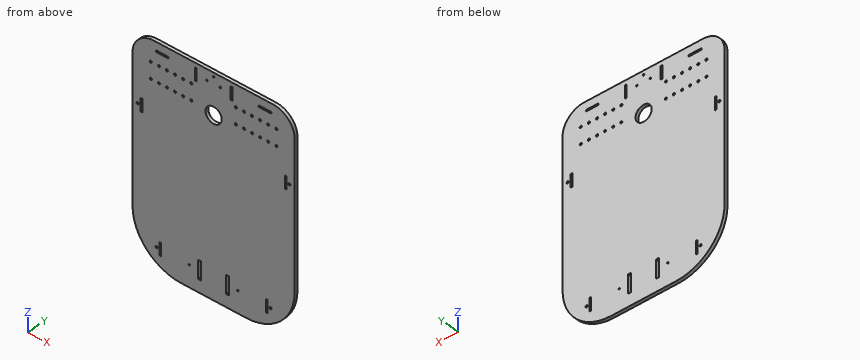
Autodesk Inventor part; units mm, degrees
ref_plane "YZ Plane" through (0, 0, 0) normal (1, 0, 0) x (0, 1, 0)
ref_plane "XZ Plane" through (0, 0, 0) normal (0, 1, 0) x (-1, 0, 0)
ref_plane "XY Plane" through (0, 0, 0) normal (0, 0, 1) x (1, 0, 0)
sketch "Sketch1" plane through (0, 0, 0) normal (0, 1, 0) x (-1, 0, 0)
  line L0 (150, 200) -> (-150, 200)
  line L1 (-150, 200) -> (-150, -200)
  line L2 (-150, -200) -> (150, -200)
  line L3 (150, -200) -> (150, 200)
  line L4 (150, 200) -> (-150, -200) construction
  line L5 (-150, 200) -> (150, -200) construction
  point P0 (0, 0)
  dimension "d0" = 300
  dimension "d1" = 400
extrude "Extrusion1" add sketch "Sketch1" along normal blind 6
sketch "Sketch2" plane through (0, 6, 0) normal (0, 1, 0) x (1, 0, 0)
  line L0 (116.2, -158) -> (86.2, -158) construction
  line L1 (86.2, -162) -> (116.2, -162) construction
  arc A0 (86.2, -158) -> (86.2, -162) centre (86.2, -160) ccw construction
  arc A1 (116.2, -162) -> (116.2, -158) centre (116.2, -160) ccw construction
  line L2 (86.2, -132) -> (116.2, -132) construction
  line L3 (116.2, -128) -> (86.2, -128) construction
  arc A2 (116.2, -132) -> (116.2, -128) centre (116.2, -130) ccw construction
  arc A3 (86.2, -128) -> (86.2, -132) centre (86.2, -130) ccw construction
  line L4 (-116.2, -162) -> (-86.2, -162) construction
  line L5 (-86.2, -158) -> (-116.2, -158) construction
  arc A4 (-116.2, -158) -> (-116.2, -162) centre (-116.2, -160) ccw construction
  arc A5 (-86.2, -162) -> (-86.2, -158) centre (-86.2, -160) ccw construction
  arc A6 (-86.2, -132) -> (-86.2, -128) centre (-86.2, -130) ccw construction
  line L6 (-86.2, -128) -> (-116.2, -128) construction
  line L7 (-116.2, -132) -> (-86.2, -132) construction
  arc A7 (-116.2, -128) -> (-116.2, -132) centre (-116.2, -130) ccw construction
  line L8 (-116.2, -162) -> (-86.2, -162) construction
  line L9 (-86.2, -158) -> (-116.2, -158) construction
  circle A8 centre (-116.2, -160) radius 2
  circle A9 centre (-116.2, -130) radius 2
  circle A10 centre (-86.2, -130) radius 2
  circle A11 centre (-101.2, -130) radius 2
  circle A12 centre (-101.2, -160) radius 2
  circle A13 centre (-86.2, -160) radius 2
  circle A14 centre (86.2, -160) radius 2
  circle A15 centre (116.2, -160) radius 2
  circle A16 centre (101.2, -160) radius 2
  circle A17 centre (101.2, -130) radius 2
  circle A18 centre (86.2, -130) radius 2
  circle A19 centre (116.2, -130) radius 2
  circle A20 centre (-71.2, -160) radius 2
  circle A21 centre (-71.2, -130) radius 2
  circle A22 centre (-56.2, -160) radius 2
  circle A23 centre (-56.2, -130) radius 2
  circle A24 centre (-41.2, -160) radius 2
  circle A25 centre (-41.2, -130) radius 2
  circle A26 centre (71.2, -130) radius 2
  circle A27 centre (71.2, -160) radius 2
  circle A28 centre (56.2, -130) radius 2
  circle A29 centre (56.2, -160) radius 2
  circle A30 centre (41.2, -130) radius 2
  circle A31 centre (41.2, -160) radius 2
  point P0 (0, 0)
  point P1 (-71.2, -158)
  point P2 (-56.2, -158)
  point P3 (-41.2, -158)
  dimension "d4" = 15
  dimension "d5" = 15
  dimension "d6" = 15
  dimension "d7" = 15
  dimension "d17" = 15
  dimension "d24" = 15
  dimension "d29" = 15
extrude "Extrusion2" cut sketch "Sketch2" against normal blind 10
sketch "Sketch4" plane through (0, 6, 0) normal (0, 1, 0) x (1, 0, 0)
  circle A0 centre (0, -125) radius 15
  line L0 (-150, -200) -> (150, -200)
  line L1 (-150, 200) -> (-150, -200)
  point P0 (0, 0)
  dimension "d30" = 30
  dimension "d31" = 75
  dimension "d32" = 150
extrude "Extrusion4" cut sketch "Sketch4" against normal blind 10
sketch "Sketch5" plane through (0, 6, 0) normal (0, 1, 0) x (1, 0, 0)
  line L0 (28.9, 177) -> (28.9, 143)
  line L1 (22.9, 143) -> (22.9, 177)
  line L2 (28.9, 177) -> (22.9, 177)
  line L3 (28.9, 143) -> (22.9, 143)
  line L4 (-22.9, 177) -> (-22.9, 143)
  line L5 (-28.9, 143) -> (-28.9, 177)
  line L6 (-28.9, 177) -> (-22.9, 177)
  line L7 (-28.9, 143) -> (-22.9, 143)
  point P0 (0, 0)
extrude "Extrusion5" cut sketch "Sketch5" against normal blind 10
sketch "Sketch6" plane through (0, 6, 0) normal (0, 1, 0) x (1, 0, 0)
  circle A0 centre (45, 160) radius 1.5
  circle A1 centre (-45, 160) radius 1.5
  point P0 (0, 0)
extrude "Extrusion6" cut sketch "Sketch6" against normal blind 10
fillet "Fillet1" radius 40 2 edges at (-150, 3, 200) (150, 3, 200)
fillet "Fillet2" radius 90 2 edges at (150, 3, -200) (-150, 3, -200)
sketch "Sketch7" plane through (0, 6, 0) normal (0, 1, 0) x (1, 0, 0)
  line L0 (-34.75, -192) -> (-34.75, -168)
  line L1 (-34.75, -168) -> (-31.75, -168)
  line L2 (-31.75, -192) -> (-31.75, -168)
  line L3 (-34.75, -192) -> (-31.75, -192)
  line L4 (31.75, -192) -> (31.75, -168)
  line L5 (31.75, -168) -> (34.75, -168)
  line L6 (34.75, -192) -> (34.75, -168)
  line L7 (31.75, -192) -> (34.75, -192)
  point P0 (0, 0)
extrude "Extrusion7" cut sketch "Sketch7" against normal blind 10
sketch "Sketch8" plane through (0, 6, 0) normal (0, 1, 0) x (1, 0, 0)
  circle A0 centre (12.5, -180) radius 1.5
  circle A1 centre (0, -192.5) radius 1.5
  circle A2 centre (-12.5, -180) radius 1.5
  point P0 (0, 0)
extrude "Extrusion8" cut sketch "Sketch8" against normal blind 10
sketch "Sketch9" plane through (0, 6, 0) normal (0, 1, 0) x (1, 0, 0)
  line L0 (-110, -200) -> (110, -200)
  line L1 (150, -160) -> (150, 110)
  line L2 (-150, 110) -> (-150, -160)
  line L3 (60, 200) -> (-60, 200)
  line L4 (0, -200) -> (0, 200) construction
  line L5 (60, 200) -> (-60, 200) construction
  line L6 (83, -185) -> (107, -185)
  line L7 (83, -185) -> (83, -182)
  line L8 (107, -182) -> (83, -182)
  line L9 (107, -185) -> (107, -182)
  line L10 (132, -63) -> (132, -87)
  line L11 (132, -63) -> (135, -63)
  line L12 (135, -87) -> (135, -63)
  line L13 (132, -87) -> (135, -87)
  line L14 (97, 172) -> (97, 148)
  line L15 (97, 172) -> (100, 172)
  line L16 (100, 148) -> (100, 172)
  line L17 (97, 148) -> (100, 148)
  line L18 (-83, -185) -> (-107, -185)
  line L19 (-83, -185) -> (-83, -182)
  line L20 (-107, -182) -> (-83, -182)
  line L21 (-107, -185) -> (-107, -182)
  line L22 (-132, -63) -> (-132, -87)
  line L23 (-132, -63) -> (-135, -63)
  line L24 (-135, -87) -> (-135, -63)
  line L25 (-132, -87) -> (-135, -87)
  line L26 (-97, 172) -> (-97, 148)
  line L27 (-97, 172) -> (-100, 172)
  line L28 (-100, 148) -> (-100, 172)
  line L29 (-97, 148) -> (-100, 148)
  point P0 (0, 0)
extrude "Extrusion9" cut sketch "Sketch9" against normal blind 10
sketch "Sketch10" plane through (0, 6, 0) normal (0, 1, 0) x (1, 0, 0)
  line L0 (135, -63) -> (135, -87) construction
  line L1 (100, 172) -> (100, 148) construction
  circle A0 centre (140.5, -75) radius 4.5 construction
  circle A1 centre (140.5, -75) radius 2
  circle A2 centre (105.5, 160) radius 4.5 construction
  circle A3 centre (105.5, 160) radius 2
  line L2 (-110, -200) -> (110, -200)
  line L3 (60, 200) -> (-60, 200)
  line L4 (0, -200) -> (0, 200) construction
  circle A4 centre (-140.5, -75) radius 4.5 construction
  circle A5 centre (-140.5, -75) radius 2
  circle A6 centre (-105.5, 160) radius 4.5 construction
  circle A7 centre (-105.5, 160) radius 2
  point P0 (0, 0)
  dimension "d47" = 9
  dimension "d48" = 12
  dimension "d50" = 5.5
  dimension "d51" = 4
  dimension "d52" = 9
  dimension "d53" = 12
  dimension "d54" = 5.5
  dimension "d55" = 4
extrude "Extrusion10" cut sketch "Sketch10" against normal blind 10
properties part number "Base"
For this review, take the finished solid that the model builds, in its own axes (mm). Round coordinates to 2 decimals unless told otherwise and drop trailing zeros.
1) Insertion check: pin 1 Ø0.9 at (x, y) = (98, 2.5) entering from -Z; pin 2 Ø1.5 at (y, z) = (4, 183) entering from +X; pin 3 Ø3.5 at (x, z) = (-116.2, 160) entering from -Y; pin 4 Ø1.8 at (y, z) = (2, -159) entering from -X. Each pin has a flat end and moves straight along its axis. Give the tip position at first contact, or say it passes through.
Answer below:
pin 1: stops at z = -191.79
pin 2: stops at x = 143.24
pin 3: passes through
pin 4: stops at x = -136.07
2) For line 1 along Z through (x, y) = (56.2, 2.25); line 2 along Z through (x, y) = (0, 3.85); line 3 along X through (y, z) = (4.25, 125), list the stretches that pass through material, from the lowest coordinate up.
Answer below:
line 1: z = -200 to 128, 132 to 158, 162 to 200
line 2: z = -200 to 110, 140 to 191, 194 to 200
line 3: x = -150 to -15, 15 to 150
3) Take a section at A-A on y = 3.9. State how many separate pieces and enclosed holes the cut face has, then the cut area to 3 significant figures.
Answer below:
separate pieces: 1
enclosed holes: 44
area: 114,000 mm2
